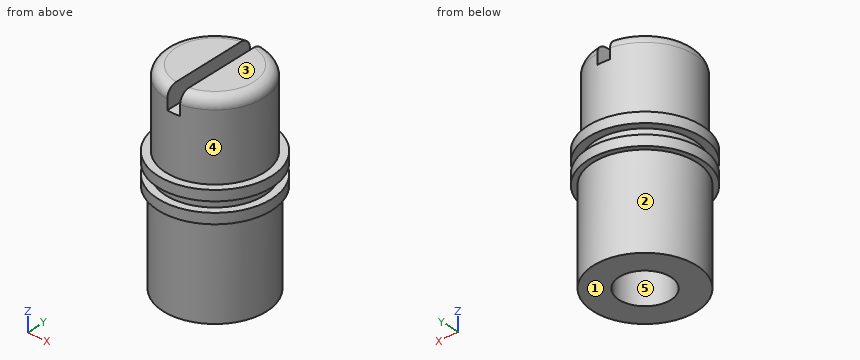
```python
from build123d import *

# Parameters (mm, degrees)
SKETCH1_R           = 9.5
BOSS_EXTRUDE1_DEPTH = 19
SKETCH1_5_R         = 10
BOSS_EXTRUDE4_DEPTH = 20
BOSS_EXTRUDE2_START = 4
SKETCH1_3_R         = 11
SKETCH1_3_R_2       = 10
SKETCH1_3_R_3       = 9.5
BOSS_EXTRUDE2_DEPTH = 2
SKETCH1_4_R         = 11
SKETCH1_4_R_2       = 10
BOSS_EXTRUDE3_DEPTH = 2
FILLET1_R           = 2
CUT_EXTRUDE3_START  = -4
CUT_EXTRUDE3_DEPTH  = 4
SKETCH6_R           = 5
CUT_EXTRUDE4_DEPTH  = 25


with BuildPart() as part:
    # Sketch1 → Boss-Extrude1 (new body)
    with BuildSketch(Plane.XY):
        Circle(SKETCH1_R)
    extrude(amount=BOSS_EXTRUDE1_DEPTH)

    # Sketch1_5 → Boss-Extrude4 (add)
    with BuildSketch(Plane.XY):
        Circle(SKETCH1_5_R)
    extrude(amount=-BOSS_EXTRUDE4_DEPTH)

    # Sketch1_3 → Boss-Extrude2 (add)
    # profile 1 of 2: a face of its own
    with BuildSketch(Plane.XY.offset(BOSS_EXTRUDE2_START)):
        Circle(SKETCH1_3_R)
        Circle(SKETCH1_3_R_2, mode=Mode.SUBTRACT)
    # profile 2 of 2: a face of its own
    with BuildSketch(Plane.XY.offset(BOSS_EXTRUDE2_START)):
        Circle(SKETCH1_3_R_2)
        Circle(SKETCH1_3_R_3, mode=Mode.SUBTRACT)
    extrude(amount=-BOSS_EXTRUDE2_DEPTH)

    # Sketch1_4 → Boss-Extrude3 (add)
    with BuildSketch(Plane.XY):
        Circle(SKETCH1_4_R)
        Circle(SKETCH1_4_R_2, mode=Mode.SUBTRACT)
    extrude(amount=-BOSS_EXTRUDE3_DEPTH)

    # Fillet1
    fillet1_edges = [part.edges().sort_by_distance(p)[0] for p in [
        (-9.5, 0, 19),
    ]]
    fillet(fillet1_edges, radius=FILLET1_R)

    # Sketch4 → Cut-Extrude3 (cut)
    with BuildSketch(Plane.XY.offset(19).offset(CUT_EXTRUDE3_START)):
        with BuildLine():
            Line((-1.25, -9.417404101), (-1.25, 9.417404101))
            ThreePointArc((-1.25, 9.417404101), (0, 9.5), (1.25, 9.417404101))
            Line((1.25, 9.417404101), (1.25, -9.417404101))
            ThreePointArc((1.25, -9.417404101), (0, -9.5), (-1.25, -9.417404101))
        make_face()
    extrude(amount=CUT_EXTRUDE3_DEPTH, mode=Mode.SUBTRACT)

    # Sketch6 → Cut-Extrude4 (cut)
    with BuildSketch(Plane(origin=(0, 0, -20), x_dir=(-1, 0, 0), z_dir=(0, 0, -1))):
        Circle(SKETCH6_R)
    extrude(amount=-CUT_EXTRUDE4_DEPTH, mode=Mode.SUBTRACT)


solid = part.part
```
Part model, mm, in its own coordinate system. Face numbers are marked on the shaded views. A direction names the side the tool comes from. Give positions to 0.01 mm unless a question says otherwise; leave off trailing zeros. Order: outer loops, then holes, each group sorted by start corner. A loop starts at its lowest first (then second) coordinate and runs counter-clockwise, first axis right, second up. Notation, with made-up numbers: M 55,15 L 102,15 A13 ccw 102,30 Z; hole C 18.5,48.5 d5. An arc over 180 degrees is marked long. Use a Markdown table: item, result. Add a question column.
(1) Saw through at D-D, the plane z = 16. Give the cut face in (x, y), and give its area (3 significant figures).
(2) 3-axis set-ups, long thin cutter, end or side, ignore diameter. For the marked faces 1 and 2: which of +Z, -Z, +X, -X, +Y, -Y reach the whole face in a straight line?
(3) Saw through at A-A, the plane x = 0. Give the cut face in (y, z).
(4) Mould opens along Y. For the marked faces 3, 4 and 5 say: +Y half, -Y half, draft (parallel to the pull), parting line (faces both ways), or undercut.
(5) Probe line 1 along Z through (x, y) = (7.5, -6.5); line 2 along Z through (x, y) = (7.25, -7.5); line 3 along Y through (x, z) = (0, -13.5). List the from-to ranges inside material, lowest first. Write a range as [from, to].
(6) Drop flat-ended pins along their axis: P1, Ø1.5, axis at x = 5.5, z = -11, coming from the +Y side; P2, Ø1, axis at x = -3, z = -2, coming from the +Y side; P3, Ø2, axis at y = -3.5, z = 17.5, coming from the +X side. Give the stop position or say it passes through.
(7) Saw through at C-C, the plane z = 1.5. Give the cut face in (x, y), and give its area (3 significant figures).
Answer key:
| question | item | result |
|---|---|---|
| 1 | outline | M -1.25,-9.42 L -1.25,9.42 A9.5 ccw Z; M 1.25,-9.42 A9.5 ccw 1.25,9.42 Z |
| 1 | area | 236 mm^2 |
| 2 | face 1 | -Z, +X, -X, +Y, -Y |
| 2 | face 2 | -Z |
| 3 | outline | M -11,-2 L -10,-2 L -10,-20 L -5,-20 L -5,5 L 5,5 L 5,-20 L 10,-20 L 10,-2 L 11,-2 L 11,0 L 9.5,0 L 9.5,2 L 11,2 L 11,4 L 9.5,4 L 9.5,15 L -9.5,15 L -9.5,4 L -11,4 L -11,2 L -9.5,2 L -9.5,0 L -11,0 Z |
| 4 | face 3 | draft |
| 4 | face 4 | parting line |
| 4 | face 5 | undercut |
| 5 | line 1 | [-20, 0], [2, 4] |
| 5 | line 2 | [-2, 0], [2, 4] |
| 5 | line 3 | [-10, -5], [5, 10] |
| 6 | P1 | y = 8.8 |
| 6 | P2 | y = 10.71 |
| 6 | P3 | x = 9.14 |
| 7 | outline | C 0,0 d19; hole C 0,0 d10 |
| 7 | area | 205 mm^2 |
